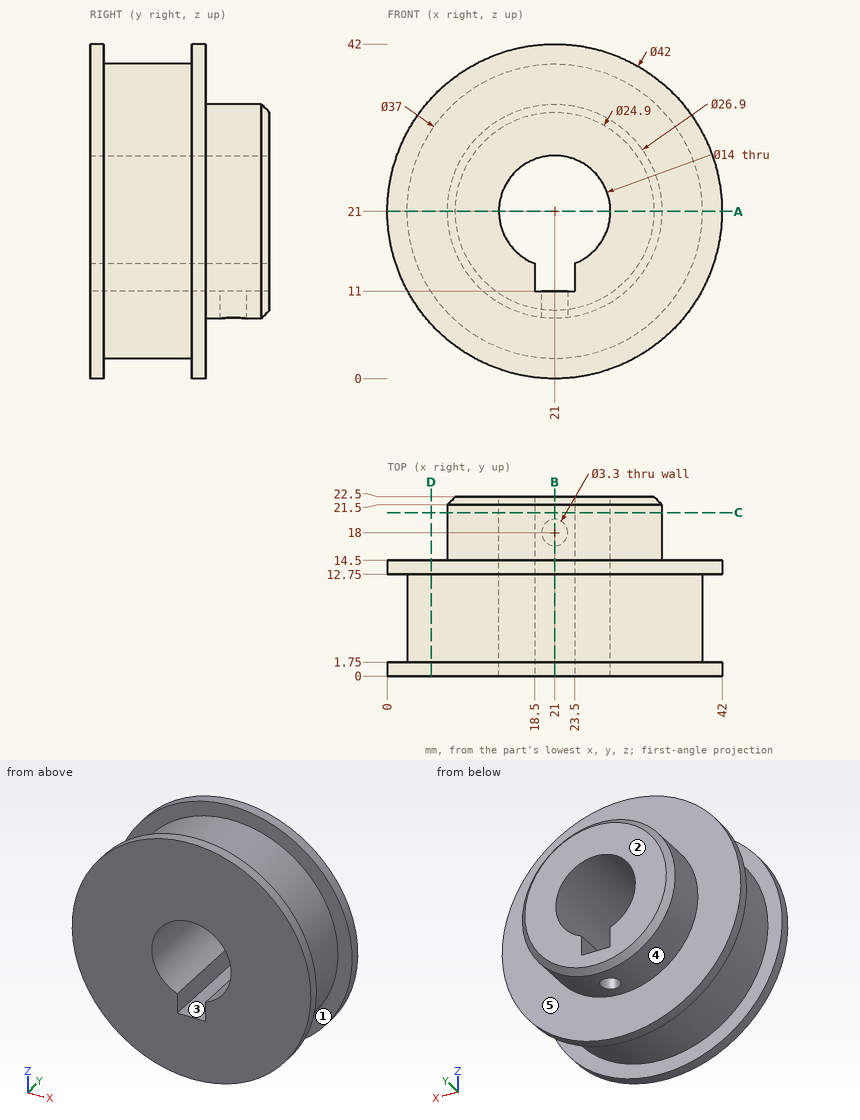
Geometry: see drawing. Coordinates: mm, zero at the bounding-box minimum. A direction names the side the tool comes from. Round coordinates to 2 decimals unless told otherwise and drop trailing zeros. Loops run counter-clockwise (first coordinate to the right, second up) from the corner with the lowest first, then second, coordinate; pieces in that order, holes last. Notation, with made-up numbers: (-27.75, 2) -> (26.25, 2) arc R17 cw to (26.25, 21) -> close; hole circle Ø5 at (26, 87). An arc over 180 degrees is marked (long way). Write each question's results on one line, items separated by ' | '.
Item 1: Set-up query: the marked faces 1 and 2. Return all of +Z, -Z, +X, -X, +Y, -Y with unobstructed straight access to the full face (end or side cutting, diameter ignored); none if empty.
Answers below:
face 1: none | face 2: +Z, -Z, +X, -X, +Y
Item 2: Line query: probe 1 along Y at (x, z) = (21, 9.65); probe 2 along X at (y, z) = (7.5, 21); probe 3 along X at (y, z) = (18, 8.85). Output: solid intervals per line, ascending. Write a range as [from, to].
Answers below:
probe 1: y = [0, 16.35], [19.65, 22.5] | probe 2: x = [2.5, 14], [28, 39.5] | probe 3: x = [15.23, 19.35], [22.65, 26.77]
Item 3: Cut plane A-A on z = 21. Return the cut outline in (x, y).
Answers below:
outline: (0, 0) -> (14, 0) -> (14, 22.5) -> (8.55, 22.5) -> (7.55, 21.5) -> (7.55, 14.5) -> (0, 14.5) -> (0, 12.75) -> (2.5, 12.75) -> (2.5, 1.75) -> (0, 1.75) -> close; (28, 0) -> (42, 0) -> (42, 1.75) -> (39.5, 1.75) -> (39.5, 12.75) -> (42, 12.75) -> (42, 14.5) -> (34.45, 14.5) -> (34.45, 21.5) -> (33.45, 22.5) -> (28, 22.5) -> close
Item 4: Pull-direction query (Z, two-part tool) for the marked faces 3, 4 and 5; classes: pulls with the +Z half, pulls with the -Z half, needs draft (parallel to the pull), parting line crosses it, or undercut.
Answers below:
face 3: undercut | face 4: parting line crosses it | face 5: needs draft
Item 5: Cut plane B-B on x = 21. Return the cut outline in (y, z), and give its area (3 significant figures).
Answers below:
outline: (0, 0) -> (1.75, 0) -> (1.75, 2.5) -> (12.75, 2.5) -> (12.75, 0) -> (14.5, 0) -> (14.5, 7.55) -> (16.35, 7.55) -> (16.35, 11) -> (0, 11) -> close; (0, 28) -> (22.5, 28) -> (22.5, 33.45) -> (21.5, 34.45) -> (14.5, 34.45) -> (14.5, 42) -> (12.75, 42) -> (12.75, 39.5) -> (1.75, 39.5) -> (1.75, 42) -> (0, 42) -> close; (19.65, 7.55) -> (21.5, 7.55) -> (22.5, 8.55) -> (22.5, 11) -> (19.65, 11) -> close | area: 374 mm²
Item 6: Cut plane C-C on y = 20.5. Return the cut outline in (x, z), and give its area (3 significant figures).
Answers below:
outline: circle Ø26.9 at (21, 21); hole (18.5, 11) -> (23.5, 11) -> (23.5, 14.46) arc R7 ccw (long way) to (18.5, 14.46) -> close | area: 399 mm²
Item 7: Cut plane D-D on x = 5.5. Return the cut outline in (y, z), and give its area (3 significant figures).
Answers below:
outline: (0, 6.83) -> (1.75, 6.83) -> (1.75, 10.9) -> (12.75, 10.9) -> (12.75, 6.83) -> (14.5, 6.83) -> (14.5, 35.17) -> (12.75, 35.17) -> (12.75, 31.1) -> (1.75, 31.1) -> (1.75, 35.17) -> (0, 35.17) -> close | area: 321 mm²
Item 8: Pin query (flat end, axial travel): pin 1 Ø11 at (x, z) = (21, 21) entering from +Y; pin 2 Ø2.5 at (x, y) = (22, 11) entering from +Z; pin 3 Ø6 at (x, z) = (29, 35.5) entering from +Y; pin 4 Ø1.7 at (y, z) = (7.5, 13.5) entering from +X. Return the tip coordinate at first contact, or that it passes through.
Answers below:
pin 1: passes through | pin 2: stops at z = 39.5 | pin 3: stops at y = 14.5 | pin 4: stops at x = 38.26
